Could you check a few things on this model? Use its own coordinates, in mm. Face numbers are marked on the shaded views. Coordinates: 2 decimals unless noted, no trailing zeros. Order: outer loops, then holes, each group sorted by start corner. A loop starts at its lowest first (then second) coordinate and runs counter-clockwise, first axis right, second up. Notation, with made-up numbers: (4, -14.75) -> (57, -14.75) arc R28 cw to (57, 19.25) -> close; hole circle Ø11 at (57, -11.75). An arc over 180 degrees is marked (long way). Return JSON: item names as keys, results as strings. Group by question number.
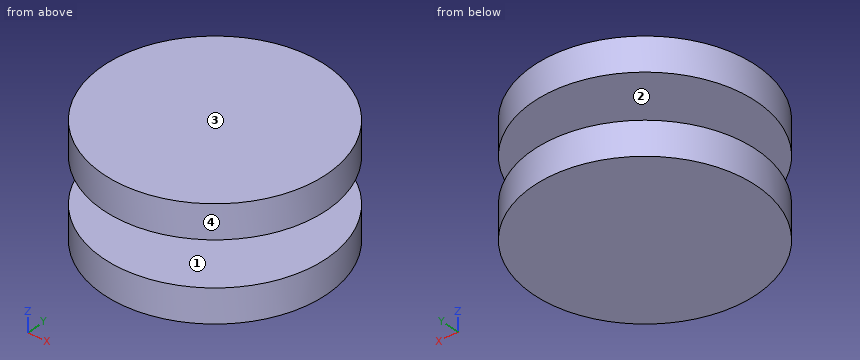
from build123d import *

# Parameters (mm, degrees)
F0_R     = 63.5
F1_DEPTH = 63.5
F2_W     = 38.1
F2_H     = 25.4


with BuildPart() as f1:
    # F0 (on Top) → F1 (new body)
    with BuildSketch(Plane.XY):
        Circle(F0_R)
    extrude(amount=F1_DEPTH)

    # F2 (on Front) → F3 (revolve, cut)
    with BuildSketch(Plane.XZ):
        with Locations((-44.45, 31.75)):
            Rectangle(F2_W, F2_H)
    revolve(axis=Axis((0, 0, 31.75), (0, 0, 1)), mode=Mode.SUBTRACT)


solid = f1.part
Q1. I'm going to push flat-ended pins straight in: pin 1 Ø10 at (x, y) = (-22, 1) entering from -Z; pin 2 Ø2 at (x, z) = (1, 44) entering from -Y; pin 3 Ø5 at (y, z) = (-45, 47) entering from +X; pin 4 Ø3 at (y, z) = (26, 48.5) entering from +X. Where does each tip first touch, or does it pass through?
Q2. I need wall thicknesses on line 1 along Z through (x, y) = (-55, -7); line 2 along Y through (x, z) = (0.5, 29); line 3 along X through (y, z) = (9, 5.5). Which ranges of each line are inside material? Lowest first, please. Write a range as from..to.
Q3. We'd pull the mould along Z, two halves only. Please class the marked faces 1, 2, 3 and 4: pulls with the +Z half, pulls with the -Z half, needs draft (parallel to the pull), parting line crosses it, or undercut.
Q4. I want a section at C-C on x = -27. Please give me the cut outline in (y, z).
Q5. I want a section at B-B on y = -50. Please give me the cut outline in (x, z), and give its area (3 significant figures).
Q6. I want a section at A-A on x = 0. Please give me the cut outline in (y, z).
Response values:
{
 "1": {"pin 1": "stops at z = 0", "pin 2": "stops at y = -63.5", "pin 3": "stops at x = 47.18", "pin 4": "stops at x = 58.58"},
 "2": {"line 1": "z = 0..19.05, 44.45..63.5", "line 2": "y = -25.4..25.4", "line 3": "x = -62.86..62.86"},
 "3": {"face 1": "undercut", "face 2": "undercut", "face 3": "pulls with the +Z half", "face 4": "needs draft"},
 "4": {"outline": "(-57.47, 0) -> (57.47, 0) -> (57.47, 19.05) -> (-57.47, 19.05) -> close; (-57.47, 44.45) -> (57.47, 44.45) -> (57.47, 63.5) -> (-57.47, 63.5) -> close"},
 "5": {"outline": "(-39.14, 0) -> (39.14, 0) -> (39.14, 19.05) -> (-39.14, 19.05) -> close; (-39.14, 44.45) -> (39.14, 44.45) -> (39.14, 63.5) -> (-39.14, 63.5) -> close", "area": "2,980 mm²"},
 "6": {"outline": "(-63.5, 0) -> (63.5, 0) -> (63.5, 19.05) -> (25.4, 19.05) -> (25.4, 44.45) -> (63.5, 44.45) -> (63.5, 63.5) -> (-63.5, 63.5) -> (-63.5, 44.45) -> (-25.4, 44.45) -> (-25.4, 19.05) -> (-63.5, 19.05) -> close"}
}
